The figure shows three views and two pictorial views of one solid part (mm, origin at its lowest corner). Answer the questions. Coordinates: 2 decimals unless noted, no trailing zeros. Loops run counter-clockwise (first coordinate to the right, second up) from the corner with the lowest first, then second, coordinate; pieces in that order, holes last. Notation, with made-up numbers: (-14.5, 55.5) - (15.5, 55.5) arc R16 ccw to (15.5, 65.5) - close; hole circle Ø5 at (76.25, 35.5). An arc over 180 degrees is marked (long way). Write each question's results on one line, items separated by ' | '. Start each with the question number.
Item 1: Section A-A, the plane x = 19.05 is taken. Write down the section's boundary in (y, z) (1 decimal).
Item 2: Section C-C, the plane z = 19 is taken. Write down the section's boundary in (x, y) (1 decimal), plus the area to 3 significant figures.
Item 3: Consider probe 1 along X at (y, z) = (2.05, 49.05); probe 2 along X at (y, z) = (1.45, 36); probe 3 along Z at (x, y) = (134, 1.4) (1 decimal). Determine where each line is inside the solid, lowest interval first. Write a range as [from, to].
Item 4: Section D-D, the plane x = 100.5 is taken. Write down the section's boundary in (y, z) (1 decimal).
Item 5: Section B-B, the plane y = 1.2 is taken. Count the separate pieces of the cut face and the enclosed holes in it, plus the area to 3 significant figures.
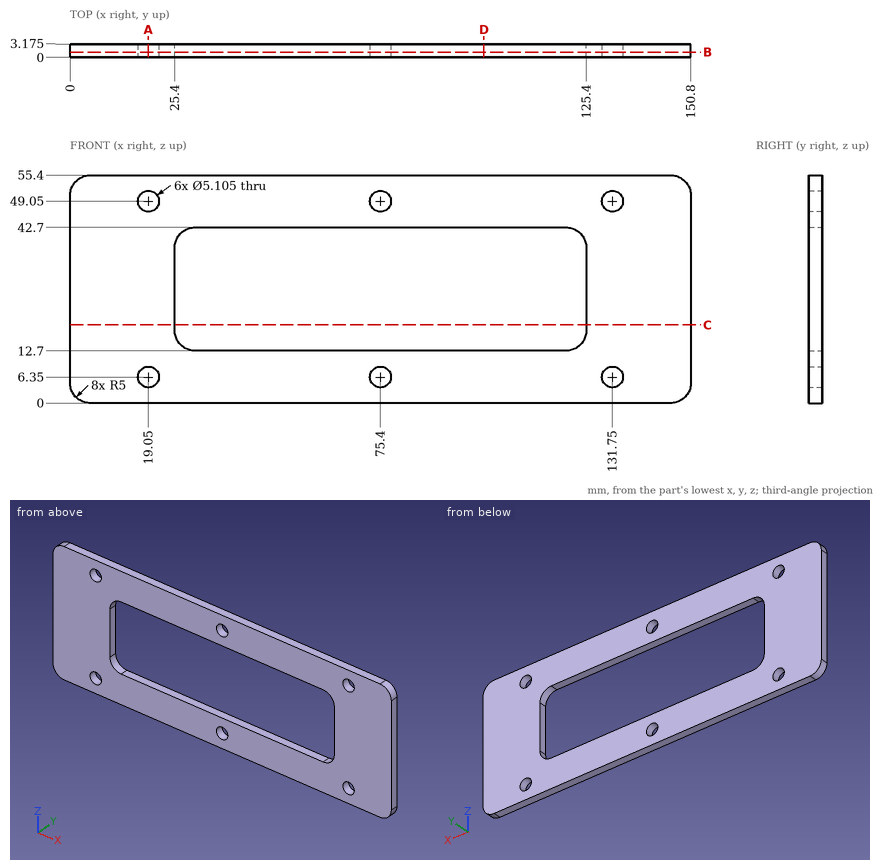
Answer key:
1) outline: (0, 0) - (3.2, 0) - (3.2, 3.8) - (0, 3.8) - close; (0, 8.9) - (3.2, 8.9) - (3.2, 46.5) - (0, 46.5) - close; (0, 51.6) - (3.2, 51.6) - (3.2, 55.4) - (0, 55.4) - close
2) outline: (0, 0) - (25.4, 0) - (25.4, 3.2) - (0, 3.2) - close; (125.4, 0) - (150.8, 0) - (150.8, 3.2) - (125.4, 3.2) - close | area: 161 mm^2
3) probe 1: x = [0, 16.5], [21.6, 72.85], [77.95, 129.2], [134.3, 150.8] | probe 2: x = [0, 25.4], [125.4, 150.8] | probe 3: z = [0, 5.1], [7.6, 47.8], [50.3, 55.4]
4) outline: (0, 0) - (3.2, 0) - (3.2, 12.7) - (0, 12.7) - close; (0, 42.7) - (3.2, 42.7) - (3.2, 55.4) - (0, 55.4) - close
5) separate pieces: 1 | enclosed holes: 7 | area: 5,230 mm^2
